from build123d import *

# Parameters (mm, degrees)
BOSS_EXTRUDE1_DEPTH = 33.45
FILLET1_R           = 10
FILLET2_R           = 20
SHELL1_START        = -80.731515082
SHELL1_OUTLINE_W    = 157.075623287
SHELL1_OUTLINE_H    = 32.25
SHELL1_DEPTH        = 38
SHELL1_START_2      = -52.731515082
SHELL1_2_DEPTH      = 99.290578512
SHELL1_START_3      = -714.702863061
SHELL1_3_DEPTH      = 127.075623287
SHELL1_4_ANGLE      = 90
CUT_EXTRUDE1_REACH  = 164.561


with BuildPart() as part:
    # Sketch1 → Boss-Extrude1 (new body)
    with BuildSketch(Plane.XY):
        with BuildLine():
            Line((46.55906343, -744.702863061), (-72.731515082, -744.702863061))
            ThreePointArc((-72.731515082, -744.702863061), (-78.388369332, -742.359717311), (-80.731515082, -736.702863061))
            Line((-80.731515082, -736.702863061), (-80.731515082, -587.627239774))
            Line((-80.731515082, -587.627239774), (-52.731515082, -587.627239774))
            Line((-52.731515082, -587.627239774), (-52.731515082, -724.702863061))
            Line((-52.731515082, -724.702863061), (46.55906343, -724.702863061))
            Line((46.55906343, -724.702863061), (46.55906343, -744.702863061))
        make_face()
    extrude(amount=BOSS_EXTRUDE1_DEPTH)

    # Fillet1
    fillet1_edges = [part.edges().sort_by_distance(p)[0] for p in [
        (-52.731515082, -724.702863061, 16.725),
    ]]
    fillet(fillet1_edges, radius=FILLET1_R)

    # Fillet2
    fillet2_edges = [part.edges().sort_by_distance(p)[0] for p in [
        (-52.731515082, -651.165051418, 33.45),
        (-49.802582894, -721.773930873, 33.45),
        (1.913774174, -724.702863061, 33.45),
    ]]
    fillet(fillet2_edges, radius=FILLET2_R - 0.0001)  # a hair under: the kernel refuses the full size

    # Shell1: read off the stored shape, not the designer's step
    # Shell1 outline → Shell1 (cut)
    with BuildSketch(Plane.YZ.offset(SHELL1_START)):
        with Locations((-666.165051418, 16.125)):
            Rectangle(SHELL1_OUTLINE_W, SHELL1_OUTLINE_H)
    extrude(amount=SHELL1_DEPTH, mode=Mode.SUBTRACT)

    # Shell1 2 outline → Shell1 2 (cut)
    with BuildSketch(Plane.YZ.offset(SHELL1_START_2)):
        with BuildLine():
            Line((-725.902863061, 0), (-725.902863061, 13.45))
            ThreePointArc((-725.902863061, 13.45), (-731.409255575, 26.743607486), (-744.702863061, 32.25))
            Line((-744.702863061, 32.25), (-744.702863061, 0))
            Line((-744.702863061, 0), (-725.902863061, 0))
        make_face()
    extrude(amount=SHELL1_2_DEPTH, mode=Mode.SUBTRACT)

    # Shell1 3 outline → Shell1 3 (add)
    with BuildSketch(Plane(origin=(0, 0, 0), x_dir=(1, 0, 0), z_dir=(0, 1, 0)).offset(SHELL1_START_3)):
        with BuildLine():
            Line((-52.731515082, -13.45), (-52.731515082, 0))
            Line((-52.731515082, 0), (-53.931515082, 0))
            Line((-53.931515082, 0), (-53.931515082, -13.45))
            ThreePointArc((-53.931515082, -13.45), (-59.437907596, -26.743607486), (-72.731515082, -32.25))
            Line((-72.731515082, -32.25), (-65.908026238, -32.25))
            ThreePointArc((-65.908026238, -32.25), (-56.353637062, -24.928898534), (-52.731515082, -13.45))
        make_face()
    extrude(amount=SHELL1_3_DEPTH)

    # Shell1 4 outline → Shell1 4 (revolve)
    with BuildSketch(Plane(origin=(-42.731515082, -714.702863061, 0), x_dir=(-1, 0, 0), z_dir=(0, 1, 0))):
        with BuildLine():
            Line((10, 13.45), (10, 0))
            Line((10, 0), (11.2, 0))
            Line((11.2, 0), (11.2, 13.45))
            ThreePointArc((11.2, 13.45), (16.706392514, 26.743607486), (30, 32.25))
            Line((30, 32.25), (23.176511156, 32.25))
            ThreePointArc((23.176511156, 32.25), (13.62212198, 24.928898534), (10, 13.45))
        make_face()
    revolve(axis=Axis((-42.731515082, -714.702863061, 0), (0, 0, 1)), revolution_arc=SHELL1_4_ANGLE)

    # Cut-Extrude1: up to this face of the body (flat: up to its plane)
    cut_extrude1_end = Plane(part.part.faces().sort_by_distance((1.913774174, -725.902863061, 6.725))[0])
    # Sketch3 → Cut-Extrude1 (cut, up to the picked face)
    with BuildSketch(Plane(origin=(0, -724.702863061, 0), x_dir=(1, 0, 0), z_dir=(0, 1, 0)), mode=Mode.PRIVATE) as cut_extrude1_sk1:
        with BuildLine():
            Line((-29.281515082, 13.45), (-6.181515082, 13.45))
            ThreePointArc((-6.181515082, 13.45), (7.268484918, 0), (-6.181515082, -13.45))
            Line((-6.181515082, -13.45), (-29.281515082, -13.45))
            ThreePointArc((-29.281515082, -13.45), (-42.731515082, 0), (-29.281515082, 13.45))
        make_face()
    cut_extrude1_tool1 = split(extrude(cut_extrude1_sk1.sketch, amount=-CUT_EXTRUDE1_REACH, mode=Mode.PRIVATE), bisect_by=cut_extrude1_end, keep=Keep.BOTH, mode=Mode.PRIVATE)
    add(cut_extrude1_tool1.solids().sort_by(Axis((-17.731515, -724.702863, 0), (0, -1, 0)))[0], mode=Mode.SUBTRACT)


solid = part.part
Design review of the part built by this model. Coordinates are the model's own, in mm. A direction names the side the tool comes from. Coordinates: 2 decimals unless noted, no trailing zeros. Loops run counter-clockwise (first coordinate to the right, second up) from the corner with the lowest first, then second, coordinate; pieces in that order, holes last. Notation, with made-up numbers: (46, 45) -> (86, 45) arc R22 ccw to (86, 75) -> close; hole circle Ø9 at (-37, -7.75). An arc over 180 degrees is marked (long way). Use a Markdown table: item, result. Add a question column.
Item 1: Clearance check with flat-ended pins moving along their axes: P1, Ø1, axis at x = -18.5, y = -725, coming from the -Z side; P2, Ø6.5, axis at x = -37.5, z = 10, coming from the -Y side; P3, Ø8, axis at y = -635, z = 11, coming from the -X side. State where each tip first meets the part, or that it passes through.
Item 2: We need section A-A, the plane z = 8. Write out the cut boundary in (x, y), and give its area (3 significant figures).
Item 3: Wall thickness on L1, parallel to Z at x = -69.5, y = -735.5; L2, parallel to Y at x = 27, z = 11; L3, parallel to X at y = -642, z = 18: over which ranges is each line inside the solid? List them lowest first. Write a range as from..to.
Item 4: Machinability: for faces 1 (the cylindrical face through (3.43, -725.29, 9.41)), 2 (the flat face through (21, -724.703, 7)), 3 (the flat face through (-53.932, -652, 7)), which of the approach directions +Z, -Z, +X, -X, +Y, -Y give a long, thin tool a straight path to every point of the face, cutting with its end or side? Answer none if there is none.
Numbers:
| question | item | result |
|---|---|---|
| 1 | P1 | stops at z = 13.45 |
| 1 | P2 | stops at y = -725.9 |
| 1 | P3 | stops at x = -54 |
| 2 | outline | (-53.93, -714.7) arc R11.2 ccw to (-42.73, -725.9) -> (-40.09, -725.9) -> (-40.09, -724.7) -> (-42.73, -724.7) arc R10 cw to (-52.73, -714.7) -> (-52.73, -587.63) -> (-53.93, -587.63) -> close; (4.63, -725.9) -> (46.56, -725.9) -> (46.56, -724.7) -> (4.63, -724.7) -> close |
| 2 | area | 226 mm^2 |
| 3 | L1 | z = 32.25..33.45 |
| 3 | L2 | y = -725.9..-724.7 |
| 3 | L3 | x = -54.49..-53.26 |
| 4 | face 1 | -Z, +Y, -Y |
| 4 | face 2 | +Z, -Z, +X, +Y |
| 4 | face 3 | -Z, -X, +Y, -Y |
